The listing builds one solid part. Answer for the finished solid, in the listing's coordinates (mm). A direction names the side the tool comes from. Round coordinates to 2 decimals unless told otherwise and drop trailing zeros. Write each loop counter-clockwise with the first axis right and the second up, starting at its lowest first coordinate (ties: lowest second). Pieces come first, ordered by that corner, then holes.
(1) Each of these flat-tipped pins is pushed along its axis until it touches: pin 1 Ø0.9 at (x, y) = (33.5, -1) entering from +Z; pin 2 Ø0.6 at (x, y) = (-33.5, -1) entering from -Z; pin 3 Ø0.9 at (y, z) = (1.5, -68.5) entering from -X. Where does it stop, or does it pass through?
(2) For faces 1 (the face through (-34.05, 0, -14)), 2 (the face through (30.68, -0.51, 65.66)), determine the directions among +Z, -Z, +X, -X, +Y, -Y from which every point of the face is accessible in a straight line to the end or side of a thin tool.
(3) A cutting plane is placed at A-A, the plane x = 19. Give the vertices of the cut face in (y, z).
(4) A cutting plane is placed at D-D, the plane z = 18.5. Give the vertices of the cut face in (x, y).
(5) The mould has two halves that part along X. Classify faces 3 (the face through (0, 0, 69.15)), 4 (the face through (0, -1, 68)), 5 (the face through (34.05, 0, -1)): +X half, -X half, draft (parallel to the pull), parting line (faces both ways), or undercut.
(6) A cutting plane is placed at C-C, the plane z = 44. Give the vertices of the cut face in (x, y).
(7) A cutting plane is placed at B-B, the plane x = -21. Give the vertices of the cut face in (y, z), and give its area (3 significant figures).
(8) Find the intervals of material crossed by probe 1 along Z at (x, y) = (25, -1.75); probe 2 along X at (y, z) = (-1, 16); probe 3 along X at (y, z) = (4.75, 59.5), in increasing order.
from build123d import *

# Parameters (mm, degrees)
F0_W      = 68.1
F0_H      = 138.3
F1_DEPTH  = 5.08
F2_R      = 8.93259
F3_T      = -1.15
F4_W      = 24.09836
F4_H      = 13.196725
F5_DEPTH  = 12.5
F6_W      = 48.097777
F6_H      = 7.753484
F7_DEPTH  = 12.5
F8_W      = 10.118616
F8_H      = 41.666549
F9_DEPTH  = 12.5
F10_W     = 6.856616
F10_H     = 19.977162
F11_DEPTH = 12.5


with BuildPart() as f1:
    # F0 (on Front) → F1 (new body, symmetric)
    with BuildSketch(Plane.XZ):
        Rectangle(F0_W, F0_H)
    extrude(amount=F1_DEPTH, both=True)

    # F2
    f2_edges = [f1.edges().sort_by_distance(p)[0] for p in [
        (-34.05, 0, 69.15),
        (34.05, 0, 69.15),
        (34.05, 0, -69.15),
        (-34.05, 0, -69.15),
    ]]
    fillet(f2_edges, radius=F2_R)

    # F3
    f3_openings = [f1.faces().sort_by_distance(p)[0] for p in [
        (0, -5.08, 0),
    ]]
    offset(amount=F3_T, openings=f3_openings)

    # F4 (on face) → F5 (cut, symmetric)
    with BuildSketch(Plane.XZ):
        with Locations((15.348363, 59.815576)):
            Rectangle(F4_W, F4_H)
    extrude(amount=F5_DEPTH, both=True, mode=Mode.SUBTRACT)

    # F6 (on face) → F7 (cut, symmetric)
    with BuildSketch(Plane(origin=(0, 0, -69.15), x_dir=(1, 0, 0), z_dir=(0, 0, -1))):
        with Locations((0.003194, 0.064824)):
            Rectangle(F6_W, F6_H)
    extrude(amount=F7_DEPTH, both=True, mode=Mode.SUBTRACT)

    # F8 (on face) → F9 (cut, symmetric)
    with BuildSketch(Plane(origin=(-34.05, 0, 0), x_dir=(0, -1, 0), z_dir=(-1, 0, 0))):
        with Locations((3.675346, 37.227889)):
            Rectangle(F8_W, F8_H)
    extrude(amount=F9_DEPTH, both=True, mode=Mode.SUBTRACT)

    # F10 (on face) → F11 (cut, symmetric)
    with BuildSketch(Plane.YZ.offset(34.05)):
        with Locations((-1.651692, 39.359077)):
            Rectangle(F10_W, F10_H)
    extrude(amount=F11_DEPTH, both=True, mode=Mode.SUBTRACT)


solid = f1.part
Solutions:
1. pin 1: stops at z = 64.32
1. pin 2: stops at z = -64.02
1. pin 3: stops at x = -29.41
2. face 1: +Z, -Z, -X, +Y, -Y
2. face 2: -Y
3. outline: (-5.08, -69.15) - (-3.94, -69.15) - (-3.94, -68) - (-5.08, -68) - close; (-5.08, 68) - (3.93, 68) - (3.93, 66.41) - (5.08, 66.41) - (5.08, 69.15) - (-5.08, 69.15) - close; (3.81, -69.15) - (5.08, -69.15) - (5.08, 53.22) - (3.93, 53.22) - (3.93, -68) - (3.81, -68) - close
4. outline: (-34.05, 1.38) - (-32.9, 1.38) - (-32.9, 3.93) - (32.9, 3.93) - (32.9, -5.08) - (34.05, -5.08) - (34.05, 5.08) - (-34.05, 5.08) - close
5. face 3: draft
5. face 4: undercut
5. face 5: +X half
6. outline: (-34.05, 1.38) - (-32.9, 1.38) - (-32.9, 3.93) - (32.9, 3.93) - (32.9, 1.78) - (34.05, 1.78) - (34.05, 5.08) - (-34.05, 5.08) - close
7. outline: (-5.08, -69.15) - (-3.94, -69.15) - (-3.94, -68) - (-5.08, -68) - close; (-5.08, 68) - (3.93, 68) - (3.93, -68) - (3.81, -68) - (3.81, -69.15) - (5.08, -69.15) - (5.08, 69.15) - (-5.08, 69.15) - close
7. area: 171 mm2
8. probe 1: z = -69.15 to -68, 68 to 69.15
8. probe 2: x = -34.05 to -32.9, 32.9 to 34.05
8. probe 3: x = -34.05 to 3.3, 27.4 to 34.05
